from build123d import *

# Parameters (mm, degrees)
F1_DEPTH = 5.08
F2_W     = 8.722898
F2_H     = 5.715
F3_DEPTH = 7.62
F4_R     = 1.31726
F5_DEPTH = 12.7


with BuildPart() as f1:
    # F0 (on Front) → F1 (new body)
    with BuildSketch(Plane.XZ):
        with BuildLine():
            ThreePointArc((-37.749078, 0), (-23.884625, -30.892331), (0, -54.894079))
            ThreePointArc((0, -54.894079), (23.167985, -30.63179), (36.846712, 0))
            Line((36.846712, 0), (36.846712, 22.108026))
            Line((36.846712, 22.108026), (-37.749078, 22.108026))
            Line((-37.749078, 22.108026), (-37.749078, 21.205658))
            Line((-37.749078, 21.205658), (-37.749078, 0))
        make_face()
    extrude(amount=F1_DEPTH)

    # F2 (on face) → F3 (join)
    with BuildSketch(Plane(origin=(0, 0, 0), x_dir=(-1, 0, 0), z_dir=(0, 1, 0))):
        Rectangle(F2_W, F2_H)
    extrude(amount=F3_DEPTH)

    # F4 (on face) → F5 (join)
    with BuildSketch(Plane(origin=(0, 0, -2.8575), x_dir=(1, 0, 0), z_dir=(0, 0, -1))):
        with Locations((0, -6.087864)):
            Circle(F4_R)
    extrude(amount=F5_DEPTH)


solid = f1.part
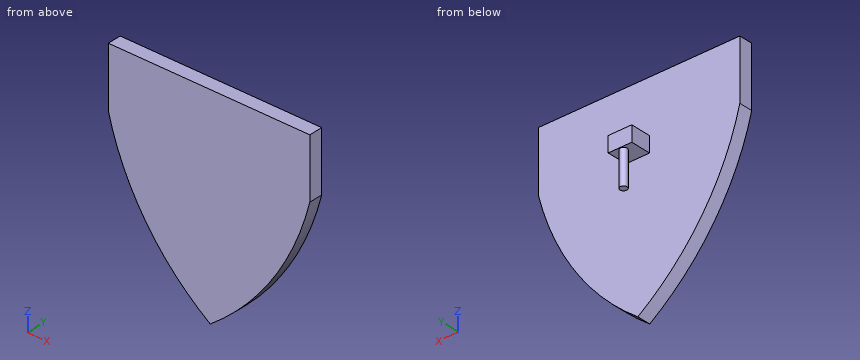
Part model, mm, in its own coordinate system. Give positions to 0.01 mm unless a question says otherwise; leave off trailing zeros. Write each loop counter-clockwise with the first axis right and the second up, starting at its lowest first coordinate (ties: lowest second). Pieces come first, ordered by that corner, then holes.
1) Cut at A-A on z = -11.5. Write the cut outline in (x, y), then the cut area to 3 significant figures.
Resolved:
outline: (-34.12, -5.08) - (33.16, -5.08) - (33.16, 0) - (-34.12, 0) - close; circle Ø2.63 at (0, 6.09)
area: 347 mm2
2) Cut at B-B on y = 2.5. Write the cut outline in (x, z).
Resolved:
outline: (-4.36, -2.86) - (4.36, -2.86) - (4.36, 2.86) - (-4.36, 2.86) - close
3) Cut at C-C on x = 19.5. Write the cut outline in (y, z).
Resolved:
outline: (-5.08, -35.74) - (0, -35.74) - (0, 22.11) - (-5.08, 22.11) - close
4) Pin check, flat tips, straight feed: pin 1 (1.5 mm diameter, centred on x = 22, y = -1, fed in from -Z); pin 2 (1.7 mm diameter, centred on y = 2.5, z = -1, fed in from +X); pin 3 (3 mm diameter, centred on x = 14, z = -21, fed in from +Y). Stop position of each tip, or through.
Resolved:
pin 1: stops at z = -33.39
pin 2: stops at x = 4.36
pin 3: stops at y = 0
5) Probe L1, parallel to Y at x = -33, z = 17; L2, parallel to Z at x = 1.5, y = 3.25; L3, parallel to X at y = -1, z = -27.5. List the from-to ranges inside material, lowest first.
Resolved:
L1: y = -5.08 to 0
L2: z = -2.86 to 2.86
L3: x = -26.11 to 25.19
